Source: CAD feature listing. Evaluate the final solid. Frame: model axes, mm. A direction names the side the tool comes from. Round coordinates to 2 decimals unless told otherwise and drop trailing zeros. Order: outer loops, then holes, each group sorted by start corner. A loop starts at its lowest first (then second) coordinate and runs counter-clockwise, first axis right, second up. Notation, with made-up numbers: (58.25, 78.5) - (67.25, 78.5) arc R15 cw to (67.25, 95.5) - close; hole circle Ø1 at (57, -38.5). An arc over 180 degrees is marked (long way). Use one line per item in the form item = value. Start each with the question number.
Q1. Cut plane B-B, the plane z = 2.5. Return the cut outline in (x, y), and give its area (3 significant figures).
Q2. Cut plane A-A, the plane x = 0. Return the cut outline in (y, z).
Q3. Cut plane C-C, the plane y = 0. Return the cut outline in (x, z).
Q4. Cut plane D-D, the plane y = 13. Return the cut outline in (x, z).
Q5. Ray query, line 1 (Y direction, x = 46.1, z = 2.5); line 2 (Z direction, x = -11, y = -24.5); line 3 (Y direction, x = -2, z = -28). Return the intervals inside material, ascending. Write a range as [from, to].
Q6. Set-up query: faces 1 (the flat face through (46, 2.352, 2)), 2 (the flat face through (-42.238, 0, 2)), 3 (the flat face through (-11, 11, 0)), 4 (the cylindrical face through (44.77, 0.38, 1.31)). Return all of +Z, -Z, +X, -X, +Y, -Y with unobstructed straight access to the full face (end or side cutting, diameter ignored); none if empty.
Q7. Pin query (flat end, axial travel): pin 1 Ø5 at (x, z) = (20.5, -2) entering from +Y; pin 2 Ø0.7 at (x, z) = (-45.5, 3) entering from -Y; pin 3 Ø1.5 at (x, z) = (13.5, -14) entering from -Y. Return the tip coordinate at first contact, or that it passes through.
Q8. Draft query along Y for faces 5 (the flat face through (-47.238, 1, 1)), 6 (the cylindrical face through (-0.96, -44.99, 2.46)), 7 (the cylindrical face through (-44.77, 0.38, 3.69)), 8 (the cylindrical face through (14.985, 0.66, -14.79)). Return one class per face: released by +Y, released by -Y, zero draft, split by the parting line, or undercut.
from build123d import *

# Parameters (mm, degrees)
BOSS_EXTRUDE2_DEPTH = 5
SKETCH6_R           = 15
BOSS_EXTRUDE3_DEPTH = 30
SKETCH7_R           = 4
BOSS_EXTRUDE4_DEPTH = 6.9
SKETCH8_R           = 1.25
CUT_EXTRUDE1_DEPTH  = 5
SKETCH9_R           = 1.25
CUT_EXTRUDE2_DEPTH  = 5


with BuildPart() as part:
    # Sketch5 → Boss-Extrude2 (new body)
    with BuildSketch(Plane.XY):
        with BuildLine():
            Line((-44.938485198, 2.352136924), (-47.238485198, 2.352136924))
            Line((-47.238485198, 2.352136924), (-47.238485198, -2.352136924))
            Line((-47.238485198, -2.352136924), (-44.938485198, -2.352136924))
            ThreePointArc((-44.938485198, -2.352136924), (0, -45), (44.938485198, -2.352136924))
            Line((44.938485198, -2.352136924), (47.238485198, -2.352136924))
            Line((47.238485198, -2.352136924), (47.238485198, 2.352136924))
            Line((47.238485198, 2.352136924), (44.938485198, 2.352136924))
            ThreePointArc((44.938485198, 2.352136924), (0, 45), (-44.938485198, 2.352136924))
        make_face()
    extrude(amount=BOSS_EXTRUDE2_DEPTH)

    # Sketch6 → Boss-Extrude3 (add)
    with BuildSketch(Plane(origin=(0, 0, 0), x_dir=(-1, 0, 0), z_dir=(0, 0, -1))):
        Circle(SKETCH6_R)
    extrude(amount=BOSS_EXTRUDE3_DEPTH)

    # Sketch7 → Boss-Extrude4 (add)
    with BuildSketch(Plane(origin=(0, 0, -30), x_dir=(-1, 0, 0), z_dir=(0, 0, -1))):
        Circle(SKETCH7_R)
    extrude(amount=BOSS_EXTRUDE4_DEPTH)

    # Sketch8 → Cut-Extrude1 (cut)
    with BuildSketch(Plane(origin=(47.238485198, 0, 0), x_dir=(0, 0, -1), z_dir=(1, 0, 0))):
        with Locations((-2.5, 0)):
            Circle(SKETCH8_R)
    extrude(amount=-CUT_EXTRUDE1_DEPTH, mode=Mode.SUBTRACT)

    # Sketch9 → Cut-Extrude2 (cut)
    with BuildSketch(Plane.ZY.offset(47.238485198)):
        with Locations((2.5, 0)):
            Circle(SKETCH9_R)
    extrude(amount=-CUT_EXTRUDE2_DEPTH, mode=Mode.SUBTRACT)


solid = part.part
Completed:
q1.outline = (-47.24, -2.35) - (-44.94, -2.35) arc R45 ccw to (44.94, -2.35) - (47.24, -2.35) - (47.24, -1.25) - (42.24, -1.25) - (42.24, 1.25) - (47.24, 1.25) - (47.24, 2.35) - (44.94, 2.35) arc R45 ccw to (-44.94, 2.35) - (-47.24, 2.35) - (-47.24, 1.25) - (-42.24, 1.25) - (-42.24, -1.25) - (-47.24, -1.25) - close
q1.area = 6,360 mm2
q2.outline = (-45, 0) - (-15, 0) - (-15, -30) - (-4, -30) - (-4, -36.9) - (4, -36.9) - (4, -30) - (15, -30) - (15, 0) - (45, 0) - (45, 5) - (-45, 5) - close
q3.outline = (-47.24, 0) - (-15, 0) - (-15, -30) - (-4, -30) - (-4, -36.9) - (4, -36.9) - (4, -30) - (15, -30) - (15, 0) - (47.24, 0) - (47.24, 1.25) - (42.24, 1.25) - (42.24, 3.75) - (47.24, 3.75) - (47.24, 5) - (-47.24, 5) - (-47.24, 3.75) - (-42.24, 3.75) - (-42.24, 1.25) - (-47.24, 1.25) - close
q4.outline = (-43.08, 0) - (-7.48, 0) - (-7.48, -30) - (7.48, -30) - (7.48, 0) - (43.08, 0) - (43.08, 5) - (-43.08, 5) - close
q5.line_1 = [-2.35, -1.25], [1.25, 2.35]
q5.line_2 = [0, 5]
q5.line_3 = [-14.87, 14.87]
q6.face_1 = +Z, -Z, +X, +Y
q6.face_2 = -X
q6.face_3 = -Z
q6.face_4 = +X
q7.pin_1 = 40.79
q7.pin_2 = -2.35
q7.pin_3 = -7.9
q8.face_5 = zero draft
q8.face_6 = released by -Y
q8.face_7 = undercut
q8.face_8 = split by the parting line
